```python
from build123d import *

# Parameters (mm, degrees)
SKETCH1_R             = 14
BOSS_EXTRUDE1_DEPTH   = 1.5875
F_3_0MM_DOWEL_HOLE1_D = 3.1


with BuildPart() as part:
    # Sketch1 → Boss-Extrude1 (new body)
    with BuildSketch(Plane(origin=(0, 0, 0), x_dir=(1, 0, 0), z_dir=(0, 1, 0))):
        with Locations(Location((0, 0, 0), (0, 0, 270))):
            Circle(SKETCH1_R)
    extrude(amount=BOSS_EXTRUDE1_DEPTH)

    # Ø3.0mm Dowel Hole1 (through all)
    with Locations(Plane(origin=(0, 1.5875, 0), x_dir=(1, 0, 0), z_dir=(0, 1, 0))):
        with Locations((-5, -8.660254038), (-10, 0), (-5, 8.660254038), (5, 8.660254038), (10, 0), (5, -8.660254038)):
            Hole(F_3_0MM_DOWEL_HOLE1_D / 2)


solid = part.part
```
Check sheet for the modelled part. Datum: model origin and axes. Units: mm. Give positions to 0.01 mm unless a question says otherwise; leave off trailing zeros. Loops run counter-clockwise (first coordinate to the right, second up) from the corner with the lowest first, then second, coordinate; pieces in that order, holes last. Notation, with made-up numbers: M 18,24 L 29,24 A26 ccw 29,53 Z; hole C 56,67 d9. An arc over 180 degrees is marked long. Answer as CSV lines item,"result".
Item 1: Sectioned sample at D-D, the plane x = -5. Enter the section's corners in (y, z), then the cut area to 3 significant figures.
Reply:
outline,"M 0,-13.08 L 1.59,-13.08 L 1.59,-10.21 L 0,-10.21 Z; M 0,-7.11 L 1.59,-7.11 L 1.59,7.11 L 0,7.11 Z; M 0,10.21 L 1.59,10.21 L 1.59,13.08 L 0,13.08 Z"
area,"31.7 mm^2"
Item 2: Sectioned sample at C-C, the plane y = 0.85. Enter the section's corners in (x, z), then the cut area to 3 significant figures.
Reply:
outline,"C 0,0 d28; hole C -10,0 d3.1; hole C -5,-8.66 d3.1; hole C -5,8.66 d3.1; hole C 5,-8.66 d3.1; hole C 5,8.66 d3.1; hole C 10,0 d3.1"
area,"570 mm^2"
Item 3: Sectioned sample at B-B, the plane x = 10.5. Enter the section's corners in (y, z).
Reply:
outline,"M 0,-9.26 L 1.59,-9.26 L 1.59,-1.47 L 0,-1.47 Z; M 0,1.47 L 1.59,1.47 L 1.59,9.26 L 0,9.26 Z"
Item 4: Draft check along X on faces 1 (the face through (-13.67, 0.78, -3.03)), 2 (the face through (0, 1.588, 0)), 3 (the face through (11.23, 0.78, 0.94)). Enter one of: pulls with the +X half, pulls with the -X half, needs draft (parallel to the pull), parting line crosses it, or undercut.
Reply:
face 1,"parting line crosses it"
face 2,"needs draft"
face 3,"undercut"
Item 5: Scan lines: L1, parallel to X at y = 0.5, z = -9; L2, parallel to Z at x = -5, y = 0.9; L3, parallel to Z at x = -5.25, y = 1.1. Record each from-to range of solid material in increasing order.
Reply:
L1,"-10.72 to -6.51, -3.49 to 3.49, 6.51 to 10.72"
L2,"-13.08 to -10.21, -7.11 to 7.11, 10.21 to 13.08"
L3,"-12.98 to -10.19, -7.13 to 7.13, 10.19 to 12.98"
Item 6: Sectioned sample at A-A, the plane z = 0. Enter the section's corners in (x, y).
Reply:
outline,"M -14,0 L -11.55,0 L -11.55,1.59 L -14,1.59 Z; M -8.45,0 L 8.45,0 L 8.45,1.59 L -8.45,1.59 Z; M 11.55,0 L 14,0 L 14,1.59 L 11.55,1.59 Z"
